Here's how the part is built. I have some questions about the finished solid (model axes, mm). Coordinates: 2 decimals unless noted, no trailing zeros. Order: outer loops, then holes, each group sorted by start corner. A loop starts at its lowest first (then second) coordinate and runs counter-clockwise, first axis right, second up.
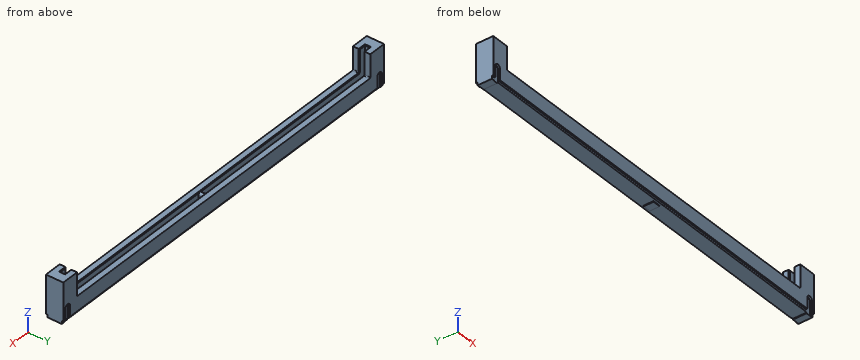
```python
from build123d import *

# Parameters (mm, degrees)
F13_DEPTH     = 3
F0_DEPTH      = 0.65
F2_W          = 2.725
F2_H          = 0.25
F3_DEPTH      = 1.3
F4_W          = 0.5
F4_H          = 1
F5_DEPTH      = 70.401
F5_DEPTH_BACK = 70.401
F6_W          = 133.75
F6_H          = 1.58
F7_DEPTH      = 11.8
F8_R          = 0.3
F9_SIZE       = 0.25
F11_DEPTH     = 1


# Not quite as in the source:
# - a pattern or mirror of a feature is missing from the dataset's text; its kind, count and spacing are read off the source's solid


with BuildPart() as f13:
    # F12 (on Front) → F13 (new body, symmetric)
    with BuildSketch(Plane.XZ):
        Polygon((-67.9, 0), (-67.9, 0.25), (1.575, 0.25), (1.575, 0), (4.3, 0), (4.3, 0.25), (67.9, 0.25), (67.9, 0), (70.4, 0), (70.4, 14.1), (64.35, 14.1), (64.35, 6.1), (-64.35, 6.1), (-64.35, 14.1), (-70.4, 14.1), (-70.4, 0), align=None)
    extrude(amount=F13_DEPTH, both=True)

    # F15: F0, F0b across plane


with BuildPart() as f0:
    # F14 (on face) → F0 (new body)
    with BuildSketch(Plane.XZ.offset(3)):
        with BuildLine():
            Line((-69.465, 4.75), (-69.465, 0))
            Line((-69.465, 0), (-67.9, 0))
            Line((-67.9, 0), (-67.9, 0.25))
            Line((-67.9, 0.25), (-67.435, 0.25))
            Line((-67.435, 0.25), (-67.435, 4.75))
            ThreePointArc((-67.435, 4.75), (-68.45, 5.765), (-69.465, 4.75))
        make_face()
    extrude(amount=-F0_DEPTH)


with BuildPart() as f0b:
    # F14 (on face) → F0, piece 2 (new body)
    with BuildSketch(Plane.XZ.offset(3)):
        with BuildLine():
            Line((67.9, 0.25), (67.9, 0))
            Line((67.9, 0), (69.465, 0))
            Line((69.465, 0), (69.465, 4.75))
            ThreePointArc((69.465, 4.75), (68.45, 5.765), (67.435, 4.75))
            Line((67.435, 4.75), (67.435, 0.25))
            Line((67.435, 0.25), (67.9, 0.25))
        make_face()
    extrude(amount=-F0_DEPTH)


with BuildPart() as f13_1:
    add(f13.part)
    add(f0.part.mirror(Plane.XZ), mode=Mode.SUBTRACT)
    add(f0b.part.mirror(Plane.XZ), mode=Mode.SUBTRACT)

    # F1: cut F0, F0b
    add(f0.part, mode=Mode.SUBTRACT)
    add(f0b.part, mode=Mode.SUBTRACT)

    # F2 (on face) → F3 (cut)
    with BuildSketch(Plane.XZ.offset(3)):
        with Locations((2.9375, 0.125)):
            Rectangle(F2_W, F2_H)
    f3 = extrude(amount=-F3_DEPTH, mode=Mode.SUBTRACT)

    # F3_copies: F3 across plane
    add(f3.mirror(Plane.ZX), mode=Mode.SUBTRACT)

    # F4 (on Right) → F5 (cut, two sides)
    with BuildSketch(Plane.YZ) as f5_sk:
        with Locations((-2.75, 0.5)):
            Rectangle(F4_W, F4_H)
        with Locations((2.75, 0.5)):
            Rectangle(F4_W, F4_H)
    extrude(amount=-F5_DEPTH, mode=Mode.SUBTRACT)
    extrude(f5_sk.sketch, amount=F5_DEPTH_BACK, mode=Mode.SUBTRACT)

    # F6 (on face) → F7 (cut)
    with BuildSketch(Plane.XY.offset(14.1)):
        Rectangle(F6_W, F6_H)
    extrude(amount=-F7_DEPTH, mode=Mode.SUBTRACT)

    # F8
    f8_edges = [f13_1.edges().sort_by_distance(p)[0] for p in [
        (-64.35, 1.895, 6.1),
        (-64.35, -1.895, 6.1),
        (64.35, 1.895, 6.1),
        (64.35, -1.895, 6.1),
    ]]
    fillet(f8_edges, radius=F8_R)

    # F9
    f9_edges = [f13_1.edges().sort_by_distance(p)[0] for p in [
        (-65.6125, 0.79, 14.1),
        (-66.875, 0, 14.1),
        (-65.6125, -0.79, 14.1),
        (-64.35, 0.79, 10.25),
        (-64.35, -0.79, 10.25),
        (65.6125, 0.79, 14.1),
        (66.875, 0, 14.1),
        (65.6125, -0.79, 14.1),
        (-64.262132, -0.79, 6.187868),
        (0, -0.79, 6.1),
        (64.262132, -0.79, 6.187868),
        (64.35, -0.79, 10.25),
        (64.35, 0.79, 10.25),
        (64.262132, 0.79, 6.187868),
        (0, 0.79, 6.1),
        (-64.262132, 0.79, 6.187868),
    ]]
    chamfer(f9_edges, length=F9_SIZE)

    # F10 (on Front) → F11 (join, symmetric)
    with BuildSketch(Plane.XZ):
        with BuildLine():
            Line((6.275, 2.3), (6.275, 5.247))
            ThreePointArc((6.275, 5.247), (5.575, 5.947), (4.875, 5.247))
            Line((4.875, 5.247), (4.875, 2.3))
            Line((4.875, 2.3), (6.275, 2.3))
        make_face()
    extrude(amount=F11_DEPTH, both=True)


solid = f13_1.part
```
Q1. Will these pins go through, and if not, where does the flat tip stop? pin 1 (1 mm diameter, centred on x = 29.5, y = -1, fed in from -Z); pin 2 (0.7 mm diameter, centred on x = -69.5, z = 0.5, fed in from -Y); pin 3 (1.6 mm diameter, centred on x = 14, y = 2, fed in from +Z); pin 4 (3.5 mm diameter, centred on x = 38, z = 8.5, fed in from -Y).
Q2. I need wall thicknesses on L1, parallel to X at y = -1.8, z = 9.5; L2, parallel to Y at x = 58, z = 5.75; L3, parallel to X at y = 0.75, z = 9.5 (3 decimals). Which ranges of each line are inside material? Lowest first, please.
Q3. If we section it at A-A on z = 10.75: Write out the boundary of the cut face in (x, y) (3 decimals), then the cut area to 3 significant figures.
Q4. If we section it at B-B on x = -9: Write out the boundary of the cut face in (y, z), then the cut area to 3 significant figures.
Reply:
1. pin 1: stops at z = 0.25
1. pin 2: stops at y = -2.5
1. pin 3: stops at z = 6.1
1. pin 4: passes through
2. L1: x = -70.4 to -64.35, 64.35 to 70.4
2. L2: y = -3 to -0.79, 0.79 to 3
2. L3: x = -70.4 to -66.875, 66.875 to 70.4
3. outline: (-70.4, -3) - (-64.35, -3) - (-64.35, -1.04) - (-64.6, -0.79) - (-66.875, -0.79) - (-66.875, 0.79) - (-64.6, 0.79) - (-64.35, 1.04) - (-64.35, 3) - (-70.4, 3) - close; (64.35, -3) - (70.4, -3) - (70.4, 3) - (64.35, 3) - (64.35, 1.04) - (64.6, 0.79) - (66.875, 0.79) - (66.875, -0.79) - (64.6, -0.79) - (64.35, -1.04) - close
3. area: 64.5 mm2
4. outline: (-3, 1) - (-2.5, 1) - (-2.5, 0.25) - (2.5, 0.25) - (2.5, 1) - (3, 1) - (3, 6.1) - (1.04, 6.1) - (0.79, 5.85) - (0.79, 2.3) - (-0.79, 2.3) - (-0.79, 5.85) - (-1.04, 6.1) - (-3, 6.1) - close
4. area: 28.3 mm2
